Autodesk Inventor part; units mm, degrees
ref_plane "Work Plane1" through (0, 0, 10) normal (0, 0, 1) x (1, 0, 0)
ref_plane "YZ Plane" through (0, 0, 0) normal (1, 0, 0) x (0, 1, 0)
ref_plane "XZ Plane" through (0, 0, 0) normal (0, 1, 0) x (-1, 0, 0)
ref_plane "Work Plane1" through (0, 0, 10) normal (0, 0, 1) x (1, 0, 0)
sketch "Sketch1" plane through (0, 0, 10) normal (0, 0, 1) x (1, 0, 0)
  line L0 (-4.0299, -0.3538) -> (-2.2322, 1.4439) construction
  arc A0 (-1.4439, 2.2322) -> (-2.2322, 1.4439) centre (-0.9299, 0.9299) ccw construction
  line L1 (-1.4439, 2.2322) -> (0.3538, 4.0299) construction
  line L2 (-37.8299, 42.8299) -> (-37.8299, 37.8299) construction
  line L3 (-37.8299, 37.8299) -> (-42.9208, 37.8299) construction
  line L4 (-37.8299, 42.2137) -> (-37.8299, 45.8299) construction
  line L5 (-37.8299, 45.8299) -> (-4.0299, 45.8299) construction
  line L6 (-4.0299, 45.8299) -> (-4.0299, 42.2137) construction
  line L7 (-4.0299, 4.0299) -> (0.3538, 4.0299)
  circle A1 centre (-20.9299, 20.9299) radius 17.5
  line L8 (-20.9299, 58.9723) -> (17.1124, 20.9299) construction
  line L9 (17.1124, 20.9299) -> (-20.9299, -17.1124) construction
  line L10 (-20.9299, -17.1124) -> (-58.9723, 20.9299) construction
  line L11 (-58.9723, 20.9299) -> (-20.9299, 58.9723) construction
  line L12 (-20.9299, 58.9723) -> (-20.9299, -17.1124) construction
  line L13 (17.1124, 20.9299) -> (-58.9723, 20.9299) construction
  line L14 (-20.9299, 58.9723) -> (32.8701, 58.9723) construction
  line L15 (-43.4299, 43.4299) -> (1.5701, 43.4299) construction
  line L16 (1.5701, 43.4299) -> (1.5701, -1.5701) construction
  line L17 (1.5701, -1.5701) -> (-43.4299, -1.5701) construction
  line L18 (-43.4299, -1.5701) -> (-43.4299, 43.4299) construction
  line L19 (-43.4299, 43.4299) -> (1.5701, -1.5701) construction
  line L20 (1.5701, 43.4299) -> (-43.4299, -1.5701) construction
  line L21 (-43.4299, 5.3876) -> (-43.4299, 36.4723)
  line L22 (-43.4299, 36.4723) -> (-36.4723, 43.4299)
  line L23 (-36.4723, 43.4299) -> (-5.3876, 43.4299)
  line L24 (-5.3876, 43.4299) -> (1.5701, 36.4723)
  line L25 (1.5701, 36.4723) -> (1.5701, 5.3876)
  line L26 (1.5701, 5.3876) -> (-5.3876, -1.5701)
  line L27 (-5.3876, -1.5701) -> (-36.4723, -1.5701)
  line L28 (-36.4723, -1.5701) -> (-43.4299, 5.3876)
  line L29 (-4.0299, 42.2137) -> (-37.8299, 42.2137)
  line L30 (-4.0299, -0.3538) -> (-4.0299, 4.0299)
  circle A2 centre (-20.9299, 20.9299) radius 1.5
  line L31 (-10.9299, 10.9299) -> (-30.9299, 10.9299) construction
  line L32 (-30.9299, 10.9299) -> (-30.9299, 30.9299) construction
  line L33 (-30.9299, 30.9299) -> (-10.9299, 30.9299) construction
  line L34 (-10.9299, 30.9299) -> (-10.9299, 10.9299) construction
  line L35 (-10.9299, 10.9299) -> (-30.9299, 30.9299) construction
  line L36 (-30.9299, 10.9299) -> (-10.9299, 30.9299) construction
  circle A3 centre (-30.9299, 30.9299) radius 1.4
  circle A4 centre (-30.9299, 10.9299) radius 1.4
  circle A5 centre (-10.9299, 10.9299) radius 1.4
  line L37 (-45.8299, 37.8299) -> (-42.0723, 37.8299) construction
  line L38 (-42.1723, 37.7299) -> (-45.8299, 37.7299)
  line L39 (-45.8299, 37.7299) -> (-45.8299, 4.1299)
  line L40 (-45.8299, 4.1299) -> (-42.1723, 4.1299)
  line L41 (-42.1723, 4.1299) -> (-42.1723, 37.7299)
  line L42 (-45.8299, 4.0299) -> (-42.0723, 4.0299) construction
  line L43 (-45.8299, 37.8299) -> (-42.0723, 37.8299)
  line L44 (-37.7299, 45.8299) -> (-4.1299, 45.8299)
  line L45 (-4.1299, 45.8299) -> (-4.1299, 42.1723)
  line L46 (-4.1299, 42.1723) -> (-37.7299, 42.1723)
  line L47 (-37.7299, 42.1723) -> (-37.7299, 45.8299)
  line L48 (0.4701, 37.8299) -> (0.4701, 4.0299) construction
  line L49 (0.4701, 4.0299) -> (3.9701, 4.0299) construction
  line L50 (3.9701, 37.8299) -> (3.9701, 4.0299) construction
  line L51 (0.4701, 37.8299) -> (3.9701, 37.8299) construction
  line L52 (-45.8299, -3.9701) -> (-4.0299, -3.9701) construction
  line L53 (0.3124, 37.7299) -> (3.9701, 37.7299)
  line L54 (3.9701, 37.7299) -> (3.9701, 4.1299)
  line L55 (3.9701, 4.1299) -> (0.3124, 4.1299)
  line L56 (0.3124, 4.1299) -> (0.3124, 37.7299)
  line L57 (-4.1713, -0.3538) -> (-37.7299, -0.3538)
  line L58 (-37.7299, -0.3538) -> (-37.7299, -3.9701)
  line L59 (-37.7299, -3.9701) -> (-4.1713, -3.9701)
  line L60 (-4.1713, -3.9701) -> (-4.1713, -0.3538)
  point P0 (-37.8299, 4.0299)
  dimension "d18" = 53.8
  dimension "d19" = 45
  dimension "d20" = 53.8
  dimension "d21" = 45
  dimension "d22" = 45
  dimension "d30" = 20
  dimension "d31" = 20
  dimension "d32" = 2.8
  dimension "d33" = 2.8
  dimension "d34" = 2.8
  dimension "d35" = 3
  dimension "d36" = 0.1
  dimension "d37" = 0.1
  dimension "d38" = 0.1
  dimension "d39" = 0.1
extrude "Extrusion1" add sketch "Sketch1" along normal blind 8 contours L30 L26 L57 L28 L41 L22 L46 L24 L56 L7 | L7 L26 L30 | L56 L24 L25 L26 | L26 L25 L24 L53 L54 L55 | L60 L59 L58 L57 L28 L27 L26 | L26 L27 L28 L57 | L46 L22 L29 L24 | L24 L29 L45 | L40 L39 L38 L22 L21 L28 | L28 L21 L22 L41 | L29 L22 L23 L24 | L24 L23 L22 L29 L47 L44 L45 | L47 L29 L22 | A1 | A2 | A3 | A4 | A5
sketch "Skizze4" plane through (0, 0, 18) normal (0, 0, 1) x (1, 0, 0)
  line L0 (-37.7299, 42.1723) -> (-42.1723, 37.7299)
  line L1 (-42.1723, 37.7299) -> (-45.8299, 37.7299)
  line L2 (-45.8299, 37.7299) -> (-45.8299, 4.1299) construction
  line L3 (-45.8299, 4.1299) -> (-42.1723, 4.1299)
  line L4 (-42.1723, 4.1299) -> (-37.6885, -0.3538)
  line L5 (-37.6885, -0.3538) -> (-37.7299, -0.3538)
  line L6 (-37.7299, -0.3538) -> (-37.7299, -3.9701)
  line L7 (-37.7299, -3.9701) -> (-4.1713, -3.9701) construction
  line L8 (-4.1713, -3.9701) -> (-4.1713, -0.3538)
  line L9 (-4.1713, -0.3538) -> (0.3124, 4.1299)
  line L10 (0.3124, 4.1299) -> (3.9701, 4.1299)
  line L11 (3.9701, 4.1299) -> (3.9701, 37.7299) construction
  line L12 (3.9701, 37.7299) -> (0.3124, 37.7299)
  line L13 (0.3124, 37.7299) -> (-4.1299, 42.1723)
  line L14 (-4.1299, 42.1723) -> (-4.1299, 45.8299)
  line L15 (-4.1299, 45.8299) -> (-37.7299, 45.8299) construction
  line L16 (-37.7299, 45.8299) -> (-37.7299, 42.1723)
  line L17 (-37.9299, 46.0299) -> (-3.9299, 46.0299) construction
  line L18 (-3.9299, 46.0299) -> (-3.9299, 42.2551)
  line L19 (-3.9299, 42.2551) -> (0.3953, 37.9299)
  line L20 (0.3953, 37.9299) -> (4.1701, 37.9299)
  line L21 (4.1701, 37.9299) -> (4.1701, 3.9299) construction
  line L22 (4.1701, 3.9299) -> (0.3953, 3.9299)
  line L23 (0.3953, 3.9299) -> (-3.9713, -0.4367)
  line L24 (-3.9713, -0.4367) -> (-3.9713, -4.1701)
  line L25 (-3.9713, -4.1701) -> (-37.9299, -4.1701) construction
  line L26 (-37.9299, -4.1701) -> (-37.9299, -0.3953)
  line L27 (-37.9299, -0.3953) -> (-42.2551, 3.9299)
  line L28 (-42.2551, 3.9299) -> (-46.0299, 3.9299)
  line L29 (-46.0299, 3.9299) -> (-46.0299, 37.9299) construction
  line L30 (-46.0299, 37.9299) -> (-42.2551, 37.9299)
  line L31 (-42.2551, 37.9299) -> (-37.9299, 42.2551)
  line L32 (-37.9299, 42.2551) -> (-37.9299, 46.0299)
  line L33 (-45.8299, 37.7299) -> (-45.8299, 37.9299)
  line L34 (-4.1299, 45.8299) -> (-37.7299, 45.8299)
  line L35 (-37.7299, 45.8299) -> (-37.9299, 45.8299)
  line L36 (-4.1299, 45.8299) -> (-3.9299, 45.8299)
  line L37 (3.9701, 37.7299) -> (3.9701, 37.9299)
  line L38 (3.9701, 4.1299) -> (3.9701, 37.7299)
  line L39 (3.9701, 4.1299) -> (3.9701, 3.9299)
  line L40 (-4.1713, -3.9701) -> (-3.9713, -3.9701)
  line L41 (-37.7299, -3.9701) -> (-37.9299, -3.9701)
  line L42 (-45.8299, 4.1299) -> (-45.8299, 3.9299)
  point P0 (0, 0)
  dimension "d40" = 0.2
extrude "IM_offset" add sketch "Skizze4" against normal up to surface (8 mm away)
sketch "Sketch27" plane through (0, 0, 18) normal (0, 0, 1) x (1, 0, 0)
  line L0 (-3.9299, 45.8299) -> (-37.9299, 45.8299)
  line L1 (-37.9299, 45.8299) -> (-37.9299, 42.2551)
  line L2 (-37.9299, 42.2551) -> (-42.2551, 37.9299)
  line L3 (-42.2551, 37.9299) -> (-45.8299, 37.9299)
  line L4 (-45.8299, 37.9299) -> (-45.8299, 3.9299)
  line L5 (-42.2551, 3.9299) -> (-45.8299, 3.9299)
  line L6 (-37.9299, -0.3953) -> (-42.2551, 3.9299)
  line L7 (-37.9299, -3.9701) -> (-37.9299, -0.3953)
  line L8 (-3.9713, -3.9701) -> (-37.9299, -3.9701)
  line L9 (-3.9713, -3.9701) -> (-3.9713, -0.4367)
  line L10 (-3.9713, -0.4367) -> (0.3953, 3.9299)
  line L11 (0.3953, 3.9299) -> (3.9701, 3.9299)
  line L12 (3.9701, 3.9299) -> (3.9701, 37.9299)
  line L13 (3.9701, 37.9299) -> (0.3953, 37.9299)
  line L14 (0.3953, 37.9299) -> (-3.9299, 42.2551)
  line L15 (-3.9299, 42.2551) -> (-3.9299, 45.8299)
  circle A0 centre (-20.9299, 20.9299) radius 24.9
  circle A1 centre (-20.9299, 20.9299) radius 2.5
  point P0 (0, 0)
  dimension "d167" = 5
extrude "Extrusion22" cut sketch "Sketch27" against normal blind 10 contours A1
sketch "Sketch28" plane through (0, 0, 18) normal (0, 0, 1) x (1, 0, 0)
  circle A0 centre (-20.9299, 20.9299) radius 2.5
  circle A1 centre (-20.9299, 20.9299) radius 4
  point P0 (0, 0)
  dimension "d170" = 8
extrude "Extrusion23" cut sketch "Sketch28" against normal blind 2
properties part number "20_Cube_Insert_single_LED_holder"
Read the model definition and answer for the solid it produces. Units are mm, in the model's axes. A direction names the side the tool comes from. Coordinates: 2 decimals unless noted, no trailing zeros. Write each loop counter-clockwise with the first axis right and the second up, starting at its lowest first coordinate (ties: lowest second). Pieces come first, ordered by that corner, then holes. Notation, with made-up numbers: (81, -10.75) -> (95, -10.75) arc R8 cw to (95, -5.75) -> close; hole circle Ø8 at (-16.5, -14). An arc over 180 degrees is marked (long way). Return JSON: item names as keys, results as strings.
(1) The part is cut by section C-C on x = -38.5. Give the vertices of the cut face in (y, z) (3 decimals).
Answers below:
{"outline": "(0.175, 10) -> (41.685, 10) -> (41.685, 18) -> (0.175, 18) -> close"}
(2) The part is cut by section A-A on y = 19.5. Give the vertices of the cut face in (x, z).
Answers below:
{"outline": "(-45.83, 10) -> (-22.98, 10) -> (-22.98, 16) -> (-24.67, 16) -> (-24.67, 18) -> (-45.83, 18) -> close; (-18.88, 10) -> (3.97, 10) -> (3.97, 18) -> (-17.19, 18) -> (-17.19, 16) -> (-18.88, 16) -> close"}
(3) The part is cut by section D-D on z = 17. Give the vertices of the cut face in (x, y).
Answers below:
{"outline": "(-45.83, 3.93) -> (-42.26, 3.93) -> (-37.93, -0.4) -> (-37.93, -3.97) -> (-3.97, -3.97) -> (-3.97, -0.44) -> (0.4, 3.93) -> (3.97, 3.93) -> (3.97, 37.93) -> (0.4, 37.93) -> (-3.93, 42.26) -> (-3.93, 45.83) -> (-37.93, 45.83) -> (-37.93, 42.26) -> (-42.26, 37.93) -> (-45.83, 37.93) -> close; hole circle Ø8 at (-20.93, 20.93)"}
(4) The part is cut by section B-B on z = 14.25. Give the vertices of the cut face in (x, y), then the cut area to 3 significant figures.
Answers below:
{"outline": "(-45.83, 3.93) -> (-42.26, 3.93) -> (-37.93, -0.4) -> (-37.93, -3.97) -> (-3.97, -3.97) -> (-3.97, -0.44) -> (0.4, 3.93) -> (3.97, 3.93) -> (3.97, 37.93) -> (0.4, 37.93) -> (-3.93, 42.26) -> (-3.93, 45.83) -> (-37.93, 45.83) -> (-37.93, 42.26) -> (-42.26, 37.93) -> (-45.83, 37.93) -> close; hole circle Ø5 at (-20.93, 20.93)", "area": "2,250 mm^2"}
(5) Consider line 1 along Y through (x, z) = (0.5, 16.5); line 2 along Y through (x, z) = (-21, 13); line 3 along Y through (x, z) = (-23, 17.25). Determine where each line is inside the solid, lowest interval first. Write a range as from..to.
Answers below:
{"line 1": "3.93..37.93", "line 2": "-3.97..18.43, 23.43..45.83", "line 3": "-3.97..17.51, 24.35..45.83"}
(6) Which of the six approach directions +Z, -Z, +X, -X, +Y, -Y give full straight-line access (tool end or side, diameter ignored) to faces 4 (the flat face through (-44, 3.93, 14)), 5 (the flat face through (-44, 37.93, 14)), 6 (the flat face through (-3.93, 44, 14)), 7 (the flat face through (2, 3.93, 14)), 8 (the cylindrical face through (-17.115, 22.131, 17.014))?
Answers below:
{"face 4": "+Z, -Z, -X, -Y", "face 5": "+Z, -Z, -X, +Y", "face 6": "+Z, -Z, +X, +Y", "face 7": "+Z, -Z, +X, -Y", "face 8": "+Z"}
(7) For a pull along X with two mould halves and no side action, classify faces 1 (the flat face through (-23, 19, 16)), 2 (the flat face through (-1.798, 40.123, 14.056)), 3 (the flat face through (-16, 21, 10)) as pulls with the +X half, pulls with the -X half, needs draft (parallel to the pull), parting line crosses it, or undercut.
Answers below:
{"face 1": "undercut", "face 2": "pulls with the +X half", "face 3": "needs draft"}
(8) Each of these flat-tipped pins is pushed along its axis until it touches: P1, Ø4.5, axis at x = -20.93, y = 20.93, coming from the +Z side; P2, Ø4, axis at x = -44, z = 16, coming from the -Y side; P3, Ø1.8, axis at x = 2.5, z = 12.5, coming from the +Y side; P4, Ø3, axis at y = -2.5, z = 12, coming from the -X side. Where does it stop, or does it pass through?
Answers below:
{"P1": "through", "P2": "y = 3.67", "P3": "y = 37.93", "P4": "x = -37.93"}
